The drawing under review shows one solid part. Ordinate dimensions are in mm from its lowest x, y, z. Coordinates: 2 decimals unless noted, no trailing zeros. Order: outer loops, then holes, each group sorted by start corner. A loop starts at its lowest first (then second) coordinate and runs counter-clockwise, first axis right, second up.
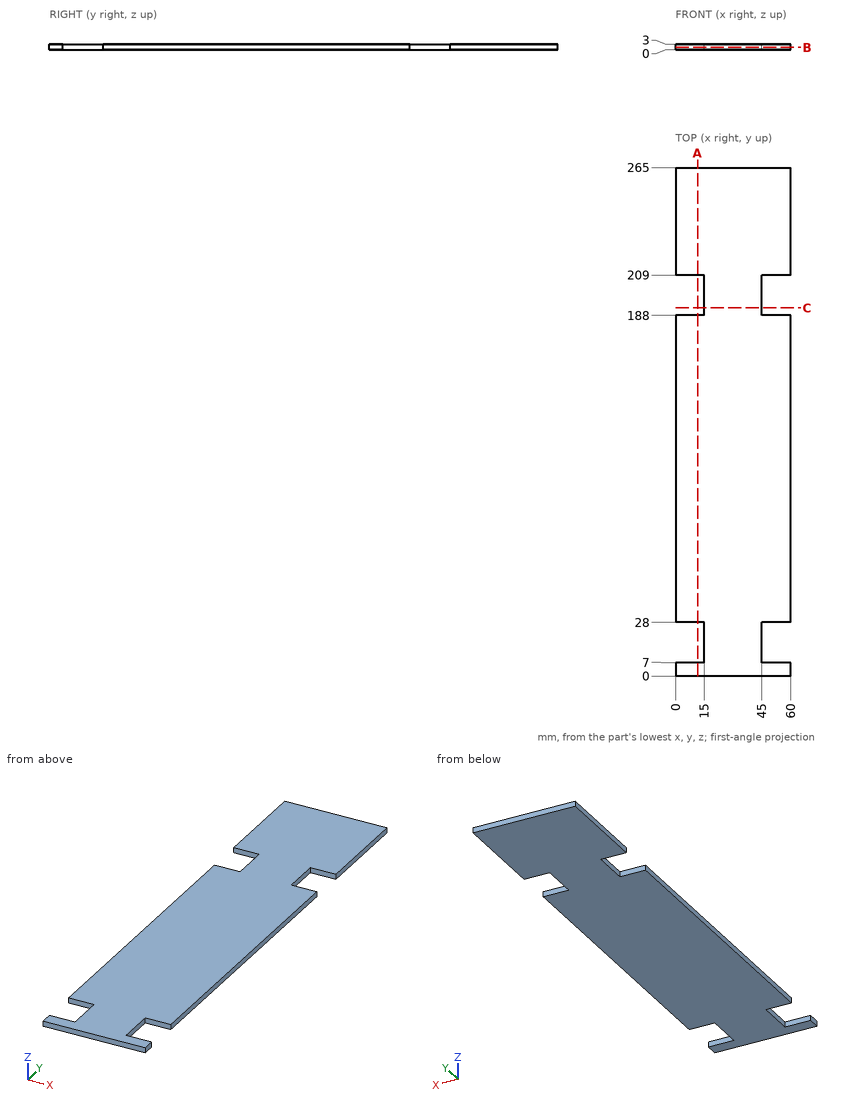
(1) Consider section B-B (z = 1.2). Give the boundary of the cut face in (x, y).
(2) Consider section A-A (x = 11.5). Give the boundary of the cut face in (y, z), then the cut area to 3 significant figures.
(3) Consider section C-C (y = 192). Give the boundary of the cut face in (x, z).
(4) Insertion check: pin 1 Ø0.9 at (x, z) = (10.5, 1) entering from -Y; pin 2 Ø1.5 at (y, z) = (13, 1) entering from +X; pin 3 Ø0.9 at (y, z) = (202, 1.5) entering from -X. Each pin has a flat end and moves straight along its axis. Give the tip position at first contact, or say it passes through.
(5) Wall thickness on line 1 (Y direction, x = 45.5, z = 1.65); line 2 (X direction, y = 14, z = 0.35): over which ranges is each line inside the solid? List them lowest first.
Findings:
1. outline: (0, 0) - (60, 0) - (60, 7) - (45, 7) - (45, 28) - (60, 28) - (60, 188) - (45, 188) - (45, 209) - (60, 209) - (60, 265) - (0, 265) - (0, 209) - (15, 209) - (15, 188) - (0, 188) - (0, 28) - (15, 28) - (15, 7) - (0, 7) - close
2. outline: (0, 0) - (7, 0) - (7, 3) - (0, 3) - close; (28, 0) - (188, 0) - (188, 3) - (28, 3) - close; (209, 0) - (265, 0) - (265, 3) - (209, 3) - close
2. area: 669 mm2
3. outline: (15, 0) - (45, 0) - (45, 3) - (15, 3) - close
4. pin 1: stops at y = 0
4. pin 2: stops at x = 45
4. pin 3: stops at x = 15
5. line 1: y = 0 to 7, 28 to 188, 209 to 265
5. line 2: x = 15 to 45
